Source: CAD feature listing. Evaluate the final solid. Frame: model axes, mm. A direction names the side the tool comes from. Coordinates: 2 decimals unless noted, no trailing zeros. Loops run counter-clockwise (first coordinate to the right, second up) from the corner with the lowest first, then second, coordinate; pieces in that order, holes last.
Item 1: Section query C-C, the plane y = -1.5. Return the cut outline in (x, z), then the cut area to 3 significant figures.
Item 2: Section query A-A, the plane y = -10. Return the cut outline in (x, z).
Item 3: Pin query (flat end, axial travel): pin 1 Ø1.2 at (x, z) = (-4.5, 1) entering from -Y; pin 2 Ø3 at (y, z) = (-2, 1.5) entering from +X; pin 3 Ø6 at (y, z) = (21, 14.5) entering from -X. Return the tip coordinate at first contact, or that it passes through.
Item 4: Section query D-D, the plane z = 46. Return the cut outline in (x, y).
Item 5: Section query B-B, the plane x = -5.5. Return the cut outline in (y, z).
Item 6: Reachability of faces 1 (the flat face through (-18.637, 0.495, 32.28)), 2 (the flat face through (0, -12.5, 1)), 3 (the flat face through (0, 12.5, 1)), 4 (the flat face through (12.63, -17.43, 27.42)) from +Z, -Z, +X, -X, +Y, -Y: full face, straight path, thin tool, end or side. Return the list, or none.
Item 7: Pull-direction query (Z, two-part tool) for faces 5 (the flat face through (-3, 0, 2.5)), 6 (the flat face through (-5.3, 17.4, 58.5)), 7 (the flat face through (12.5, 0, 1)); classes: +Z half, -Z half, draft (parallel to the pull), parting line (faces both ways), or undercut.
Item 8: Line query: probe 1 along Z at (x, y) = (-6.5, -10.5); probe 2 along Z at (x, y) = (9, 2.5); probe 3 along Y at (x, z) = (-27, 56). Output: solid intervals per line, ascending.
```python
from build123d import *

# Parameters (mm, degrees)
F0_W     = 25
F0_H     = 25
F1_DEPTH = 2.5
F5_DEPTH = 50


# Not quite as in the source:
# - a feature of the source that left no trace in its solid (it failed there, or was rolled back) is left out


with BuildPart() as f1:
    # F0 (on Top) → F1 (new body)
    with BuildSketch(Plane.XY):
        Rectangle(F0_W, F0_H)
    extrude(amount=F1_DEPTH)

    # F4 (on line) → F5 (join)
    with BuildSketch(Plane(origin=(0, 0, 0), x_dir=(0, -1, 0), z_dir=(-0.8660254038, 0, -0.5))):
        Polygon((-35.3553390593, 35.3553390593), (0, 0), (35.3553390593, 35.3553390593), (0, 70.7106781187), align=None)
    extrude(amount=-F5_DEPTH)


solid = f1.part
```
Verdict:
1. outline: (-34.61, 59.94) - (-1.44, 2.5) - (-12.5, 2.5) - (-12.5, 0) - (12.5, 0) - (12.5, 2.5) - (1.33, 2.5) - (42.55, 26.3) - (8.7, 84.94) - close
1. area: 3,450 mm2
2. outline: (-30.36, 52.58) - (-5, 8.66) - (38.3, 33.66) - (12.95, 77.58) - close; (-12.5, 0) - (12.5, 0) - (12.5, 2.5) - (-12.5, 2.5) - close
3. pin 1: stops at y = -12.5
3. pin 2: stops at x = 12.5
3. pin 3: stops at x = -10.01
4. outline: (-26.56, -17.59) - (8.96, -35.36) - (31.18, -24.25) - (31.18, 24.25) - (8.96, 35.36) - (-26.56, 17.59) - close
5. outline: (-35.36, 37.65) - (-11, 9.53) - (11, 9.53) - (35.36, 37.65) - (0, 78.47) - close; (-12.5, 0) - (12.5, 0) - (12.5, 2.5) - (-12.5, 2.5) - close
6. face 1: -X, +Y, -Y
6. face 2: -Z, +X, -X, -Y
6. face 3: -Z, +X, -X, +Y
6. face 4: +X, -Y
7. face 5: undercut
7. face 6: +Z half
7. face 7: draft
8. probe 1: z = 0 to 2.5, 11.26 to 65.77
8. probe 2: z = 0 to 2.5, 8.08 to 83.96
8. probe 3: y = -8.71 to 8.71
